```python
from build123d import *

# Parameters (mm, degrees)
SKETCH1_W           = 29
SKETCH1_H           = 28.5
BOSS_EXTRUDE1_DEPTH = 25
SKETCH2_R           = 1.3
CUT_EXTRUDE1_DEPTH  = 41.854161355
FILLET1_R           = 5
SKETCH3_W           = 23
SKETCH3_H           = 28.5
CUT_EXTRUDE2_DEPTH  = 17
SKETCH5_W           = 7
SKETCH5_H           = 18
BOSS_EXTRUDE2_DEPTH = 6
SKETCH6_W           = 7
SKETCH6_H           = 24.5
BOSS_EXTRUDE3_DEPTH = 8
SKETCH8_W           = 8
SKETCH8_H           = 26.5
BOSS_EXTRUDE4_DEPTH = 9
SKETCH9_W           = 7
SKETCH9_H           = 24.5
BOSS_EXTRUDE5_DEPTH = 8
CUT_EXTRUDE5_DEPTH  = 31
SKETCH11_W          = 20
SKETCH11_H          = 6.645872657
BOSS_EXTRUDE6_DEPTH = 5
SKETCH14_W          = 15
SKETCH14_H          = 12
CUT_EXTRUDE8_DEPTH  = 26
SKETCH15_W          = 7.764432238
SKETCH15_H          = 5.354127343
CUT_EXTRUDE9_DEPTH  = 25
SKETCH16_W          = 15
SKETCH16_H          = 4
CUT_EXTRUDE11_DEPTH = 26


with BuildPart() as part:
    # Sketch1 → Boss-Extrude1 (new body)
    with BuildSketch(Plane.XY):
        Rectangle(SKETCH1_W, SKETCH1_H)
    extrude(amount=BOSS_EXTRUDE1_DEPTH)

    # Sketch2 → Cut-Extrude1 (cut, through all)
    with BuildSketch(Plane(origin=(14.5, 0, 0), x_dir=(0, 0, -1), z_dir=(1, 0, 0))):
        with Locations(Location((-3.25, 11, 0), (0, 0, 90))):
            Circle(SKETCH2_R)
        with Locations(Location((-3.25, -11, 0), (0, 0, 90))):
            Circle(SKETCH2_R)
    extrude(amount=-CUT_EXTRUDE1_DEPTH, mode=Mode.SUBTRACT)

    # Fillet1
    fillet1_edges = [part.edges().sort_by_distance(p)[0] for p in [
        (0, -14.25, 0),
        (0, 14.25, 0),
    ]]
    fillet(fillet1_edges, radius=FILLET1_R)

    # Sketch3 → Cut-Extrude2 (cut)
    with BuildSketch(Plane(origin=(0, 0, 0), x_dir=(-1, 0, 0), z_dir=(0, 0, -1))):
        Rectangle(SKETCH3_W, SKETCH3_H)
    extrude(amount=-CUT_EXTRUDE2_DEPTH, mode=Mode.SUBTRACT)

    # Sketch5 → Boss-Extrude2 (add)
    with BuildSketch(Plane.XY.offset(25)):
        with Locations((-11, 5.25)):
            Rectangle(SKETCH5_W, SKETCH5_H)
    extrude(amount=BOSS_EXTRUDE2_DEPTH)

    # Sketch6 → Boss-Extrude3 (add)
    with BuildSketch(Plane.XY.offset(25)):
        with Locations((-4, 2)):
            Rectangle(SKETCH6_W, SKETCH6_H)
    extrude(amount=BOSS_EXTRUDE3_DEPTH)

    # Sketch8 → Boss-Extrude4 (add)
    with BuildSketch(Plane.XY.offset(25)):
        with Locations((3.5, 1)):
            Rectangle(SKETCH8_W, SKETCH8_H)
    extrude(amount=BOSS_EXTRUDE4_DEPTH)

    # Sketch9 → Boss-Extrude5 (add)
    with BuildSketch(Plane.XY.offset(25)):
        with Locations((11, 2)):
            Rectangle(SKETCH9_W, SKETCH9_H)
    extrude(amount=BOSS_EXTRUDE5_DEPTH)

    # Sketch10 → Cut-Extrude5 (cut)
    with BuildSketch(Plane(origin=(14.5, 0, 0), x_dir=(0, 0, -1), z_dir=(1, 0, 0))):
        Polygon((-33, 6.25), (-25, 14.25), (-33, 14.25), align=None)
        Polygon((-34, 5.25), (-33, 6.25), (-33, 14.25), (-34, 14.25), align=None)
    extrude(amount=-CUT_EXTRUDE5_DEPTH, mode=Mode.SUBTRACT)

    # Sketch11 → Boss-Extrude6 (add)
    with BuildSketch(Plane(origin=(14.5, 0, 0), x_dir=(0, 0, -1), z_dir=(1, 0, 0))):
        with Locations((-22, -10.927063672)):
            Rectangle(SKETCH11_W, SKETCH11_H)
    extrude(amount=BOSS_EXTRUDE6_DEPTH)

    # Sketch14 → Cut-Extrude8 (cut)
    with BuildSketch(Plane.ZY.offset(14.5)):
        with Locations((17.5, -8.25)):
            Rectangle(SKETCH14_W, SKETCH14_H)
    extrude(amount=-CUT_EXTRUDE8_DEPTH, mode=Mode.SUBTRACT)

    # Sketch15 → Cut-Extrude9 (cut)
    with BuildSketch(Plane.ZY.offset(-11.5)):
        with Locations((21.117783881, -4.927063672)):
            Rectangle(SKETCH15_W, SKETCH15_H)
    extrude(amount=-CUT_EXTRUDE9_DEPTH, mode=Mode.SUBTRACT)

    # Sketch16 → Cut-Extrude11 (cut)
    with BuildSketch(Plane.ZY.offset(14.5)):
        with Locations((17.5, -0.25)):
            Rectangle(SKETCH16_W, SKETCH16_H)
    extrude(amount=-CUT_EXTRUDE11_DEPTH, mode=Mode.SUBTRACT)


solid = part.part
```
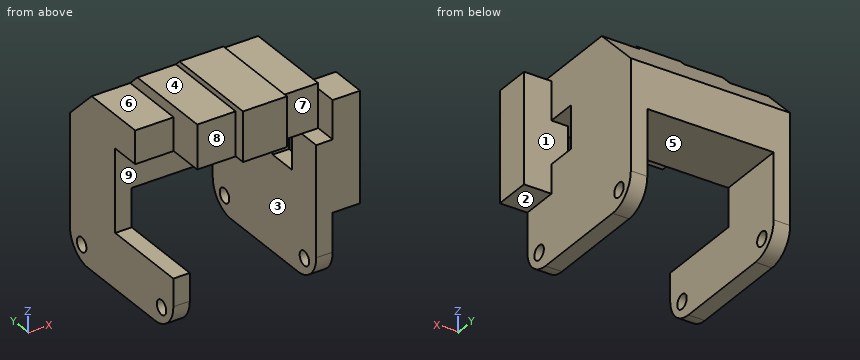
The model under review builds one solid part; all positions refer to its coordinate system, in mm. Face numbers are marked on the shaded views. A direction names the side the tool comes from. Round coordinates to 2 decimals unless told otherwise and drop trailing zeros. Order: outer loops, then holes, each group sorted by start corner. A loop starts at its lowest first (then second) coordinate and runs counter-clockwise, first axis right, second up. Notation, with made-up numbers: (23.25, -32) -> (45.25, -32) arc R26 ccw to (45.25, -10) -> close; hole circle Ø10 at (43.25, -22). An arc over 180 degrees is marked (long way). One line per item, written item: value. Start each with the question number.
Q1. Clearance check with flat-ended pins moving along their axes: pin 1 Ø2 at (x, y) = (-7.5, -11) entering from -Z; pin 2 Ø7.5 at (x, z) = (0.5, 16) entering from -Y; pin 3 Ø3.5 at (x, y) = (12.5, -5.5) entering from +Z; pin 4 Ø2.5 at (y, z) = (-11, 3.25) entering from +X. State where each tip first meets the part, or that it passes through.
Q2. Mouldability with a two-part tool opening along Z and no side actions: class the marked faces 1, 2, 3 and 4 as released by +Z, released by -Z, zero draft, split by the parting line, or undercut.
Q3. Take a section at C-C (y = -11). Write out the cut boundary in (x, z), and give its area (3 significant figures).
Q4. Wall thickness on line 1 (X direction, y = 10.5, z = 7.5); line 2 (Y direction, x = -5, z = 19); line 3 (Z direction, x = -12.8, y = -11): over which ranges is each line inside the solid? List them lowest first.
Q5. Take a section at A-A (z = 15). Write out the cut boundary in (x, y).
Q6. Machinability: for the marked faces 5, 6, 7, 8 and 9, which of the approach directions +Z, -Z, +X, -X, +Y, -Y give a long, thin tool a straight path to every point of the face, cutting with its end or side? Answer none if there is none.
Q7. Take a section at D-D (z = 27). Write out the cut boundary in (x, y), and give its area (3 significant figures).
Q8. Take a section at B-B (x = 2). Write out the cut boundary in (y, z).
Reported:
1. pin 1: stops at z = 25
1. pin 2: stops at y = 1.75
1. pin 3: stops at z = 33
1. pin 4: passes through
2. face 1: undercut
2. face 2: released by -Z
2. face 3: zero draft
2. face 4: released by +Z
3. outline: (-14.5, 0.32) -> (-11.5, 0.32) -> (-11.5, 1.95) -> (-14.5, 1.95) -> close; (-14.5, 4.55) -> (-11.5, 4.55) -> (-11.5, 10) -> (-14.5, 10) -> close; (-0.5, 25) -> (7.5, 25) -> (7.5, 34) -> (-0.5, 34) -> close; (11.5, 0.32) -> (14.5, 0.32) -> (14.5, 1.95) -> (11.5, 1.95) -> close; (11.5, 4.55) -> (14.5, 4.55) -> (14.5, 12) -> (19.5, 12) -> (19.5, 32) -> (14.5, 32) -> (14.5, 25) -> (11.5, 25) -> close
3. area: 260 mm2
4. line 1: x = -14.5 to -11.5, 11.5 to 14.5
4. line 2: y = 1.75 to 14.25
4. line 3: z = 0.32 to 1.95, 4.55 to 10
5. outline: (-14.5, 1.75) -> (-11.5, 1.75) -> (-11.5, 14.25) -> (-14.5, 14.25) -> close; (11.5, -14.25) -> (19.5, -14.25) -> (19.5, -7.6) -> (14.5, -7.6) -> (14.5, 14.25) -> (11.5, 14.25) -> close
6. face 5: -Z, +Y, -Y
6. face 6: +Z, -X, +Y, -Y
6. face 7: +Z, -Y
6. face 8: +Z, -Z, -X, -Y
6. face 9: -X, -Y
7. outline: (-14.5, -3.75) -> (-7.5, -3.75) -> (-7.5, -10.25) -> (-0.5, -10.25) -> (-0.5, -12.25) -> (7.5, -12.25) -> (7.5, -10.25) -> (14.5, -10.25) -> (14.5, -14.25) -> (19.5, -14.25) -> (19.5, -7.6) -> (14.5, -7.6) -> (14.5, 12.25) -> (-14.5, 12.25) -> close
7. area: 656 mm2
8. outline: (-12.25, 25) -> (1.75, 25) -> (1.75, 17) -> (14.25, 17) -> (14.25, 25) -> (5.25, 34) -> (-12.25, 34) -> close
